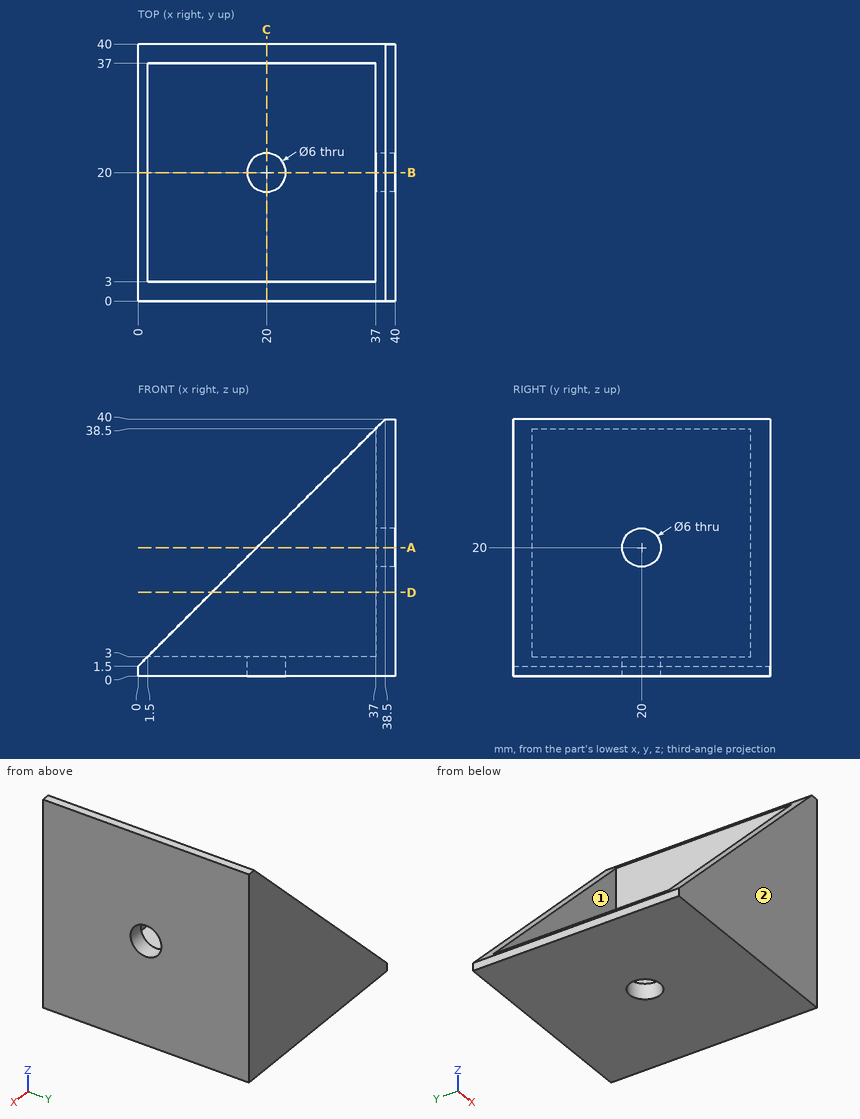
The figure shows three views and two pictorial views of one solid part (mm, origin at its lowest corner). Answer the questions. A direction names the side the tool comes from. Round coordinates to 2 decimals unless told otherwise and drop trailing zeros. Write each loop counter-clockwise with the first axis right and the second up, starting at its lowest first coordinate (ties: lowest second). Pieces come first, ordered by that corner, then holes. Notation, with made-up numbers: M 14.25,-16 L 26.25,-16 A22 ccw 26.25,21 Z; hole C -23,67 d1. An arc over 180 degrees is marked long. Use a Markdown table: item, result.
1) Straight lines are drawn through the part: line 1 along Y through (x, z) = (35, 16.5); line 2 along Y through (x, z) = (38.2, 20); line 3 along X through (y, z) = (28.5, 28.5). For each, find the intervals that lie inside material, in ascending order. Write a range as [from, to].
Answers follow:
| item | result |
|---|---|
| line 1 | y = [0, 3], [37, 40] |
| line 2 | y = [0, 17], [23, 40] |
| line 3 | x = [37, 40] |
2) The part is cut by section C-C (x = 20). Write down the section's boundary in (y, z), plus the area to 3 significant figures.
Answers follow:
| item | result |
|---|---|
| outline | M 0,0 L 17,0 L 17,3 L 3,3 L 3,21.5 L 0,21.5 Z; M 23,0 L 40,0 L 40,21.5 L 37,21.5 L 37,3 L 23,3 Z |
| area | 213 mm2 |
3) The part is cut by section B-B (y = 20). Write down the section's boundary in (x, z), plus the area to 3 significant figures.
Answers follow:
| item | result |
|---|---|
| outline | M 0,0 L 17,0 L 17,3 L 1.5,3 L 0,1.5 Z; M 23,0 L 40,0 L 40,17 L 37,17 L 37,3 L 23,3 Z; M 37,23 L 40,23 L 40,40 L 38.5,40 L 37,38.5 Z |
| area | 193 mm2 |
4) The part is cut by section D-D (z = 13). Write down the section's boundary in (x, y), plus the area to 3 significant figures.
Answers follow:
| item | result |
|---|---|
| outline | M 11.5,0 L 40,0 L 40,40 L 11.5,40 L 11.5,37 L 37,37 L 37,3 L 11.5,3 Z |
| area | 273 mm2 |
5) The part is cut by section A-A (z = 20). Write down the section's boundary in (x, y), plus the area to 3 significant figures.
Answers follow:
| item | result |
|---|---|
| outline | M 18.5,0 L 40,0 L 40,17 L 37,17 L 37,3 L 18.5,3 Z; M 18.5,37 L 37,37 L 37,23 L 40,23 L 40,40 L 18.5,40 Z |
| area | 213 mm2 |
6) A tool of negligible diameter and unlimited length cuts with its end or side. For the marked faces 1 and 2, from which of +Z, -Z, +X, -X, +Y, -Y can it reach the whole face along a straight path? Write none if from no direction.
Answers follow:
| item | result |
|---|---|
| face 1 | +Z, -X |
| face 2 | +Z, -Z, +X, -X, -Y |
7) Flat-ended cylindrical pins translate along their axes: pin 1 (2 mm diameter, centred on y = 25, z = 16.5, fed in from -X); pin 2 (6 mm diameter, centred on x = 19.5, y = 29, fed in from +Z); pin 3 (5 mm diameter, centred on y = 20, z = 20, fed in from -X). Find the tip coordinate at first contact, or state that the pin passes through.
Answers follow:
| item | result |
|---|---|
| pin 1 | stops at x = 37 |
| pin 2 | stops at z = 3 |
| pin 3 | passes through |
